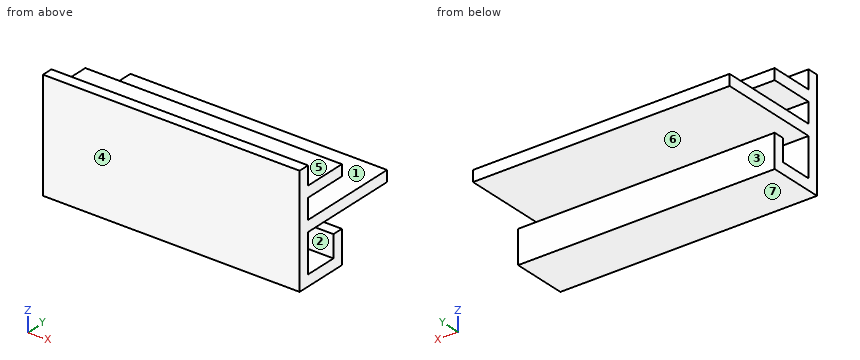
```python
from build123d import *

# Parameters (mm, degrees)
SKETCH_1_W      = 3
SKETCH_1_H      = 12
SKETCH_1_W_2    = 30
SKETCH_1_H_2    = 3
SKETCH_1_W_3    = 6
SKETCH_1_H_3    = 28
EXTRUDE_1_DEPTH = 70


with BuildPart() as part:
    # Sketch 1 → Extrude 1 (new body)
    with BuildSketch(Plane(origin=(0, 0, 0), x_dir=(0, 0, -1), z_dir=(1, 0, 0))):
        with Locations((-8.5, 7.5)):
            Rectangle(SKETCH_1_W, SKETCH_1_H)
        Rectangle(SKETCH_1_W_2, SKETCH_1_H_2)
        Polygon((15, 13.5), (12, 13.5), (12, 10.5), (12, 1.5), (15, 1.5), align=None)
        with Locations((9, 12)):
            Rectangle(SKETCH_1_W_3, SKETCH_1_H_2)
        with Locations((0, 15.5)):
            Rectangle(SKETCH_1_W, SKETCH_1_H_3)
    extrude(amount=EXTRUDE_1_DEPTH)


solid = part.part
```
CAD build for the part. Positions are in the model's coordinates, mm. Face numbers are marked on the shaded views. A direction names the side the tool comes from. Round coordinates to 2 decimals unless told otherwise and drop trailing zeros. Loops run counter-clockwise (first coordinate to the right, second up) from the corner with the lowest first, then second, coordinate; pieces in that order, holes last. Notation, with made-up numbers: M 32,77 L 53,77 A32 cw 53,107 Z; hole C -9.5,83 d8. An arc over 180 degrees is marked long. Return JSON: item names as keys, results as strings. Group by question number.
(1) Drop flat-ended pins along their axis: P1, Ø3, axis at x = 41.5, z = 5, coming from the +Y side; P2, Ø7, axis at x = 46, z = -8.5, coming from the +Y side; P3, Ø12, axis at x = 42, y = 25.5, coming from the +Z side. Give the stop position or say it passes through.
(2) Tool access for the marked faces 1, 2 and 3: list every direction of +Z, -Z, +X, -X, +Y, -Y with a clear straight run to the whole face (end or side of a thin tool).
(3) Mould opens along Z. For the marked faces 4, 5, 6 and 7 say: +Z half, -Z half, draft (parallel to the pull), parting line (faces both ways), or undercut.
(4) Saw through at D-D, the plane z = 4.75. List the corners of the cut face in (x, y), and give its area (3 significant figures).
(5) Saw through at A-A, the plane z = -7.75. List the corners of the cut face in (x, y), and give its area (3 significant figures).
(6) Saw through at C-C, the plane x = 8. List the corners of the cut face in (y, z), and give its area (3 significant figures).
(7) Wall check: probe 1 along Z at (x, y) = (33.5, 4.5); probe 2 along Y at (x, z) = (59.5, -8.5); probe 3 along Z at (x, y) = (25.5, 16). Give the ranges that are in metal, low to high. Write a range as [from, to].
(8) Saw through at B-B, the plane y = 8. List the corners of the cut face in (x, z), and give its area (3 significant figures).
Answer list:
{
 "1": {"P1": "y = 1.5", "P2": "y = 13.5", "P3": "z = 1.5"},
 "2": {"face 1": "+X, -X, +Y", "face 2": "+X, -X", "face 3": "-Z, +X, -X, +Y"},
 "3": {"face 4": "draft", "face 5": "+Z half", "face 6": "undercut", "face 7": "-Z half"},
 "4": {"outline": "M 0,-1.5 L 70,-1.5 L 70,1.5 L 0,1.5 Z", "area": "210 mm2"},
 "5": {"outline": "M 0,-1.5 L 70,-1.5 L 70,1.5 L 0,1.5 Z; M 0,10.5 L 70,10.5 L 70,13.5 L 0,13.5 Z", "area": "420 mm2"},
 "6": {"outline": "M -1.5,-15 L 13.5,-15 L 13.5,-6 L 10.5,-6 L 10.5,-12 L 1.5,-12 L 1.5,-1.5 L 29.5,-1.5 L 29.5,1.5 L 1.5,1.5 L 1.5,7 L 13.5,7 L 13.5,10 L 1.5,10 L 1.5,15 L -1.5,15 Z", "area": "264 mm2"},
 "7": {"probe 1": "[-15, -12], [-1.5, 1.5], [7, 10]", "probe 2": "[-1.5, 1.5], [10.5, 13.5]", "probe 3": "[-1.5, 1.5]"},
 "8": {"outline": "M 0,-15 L 70,-15 L 70,-12 L 0,-12 Z; M 0,-1.5 L 70,-1.5 L 70,1.5 L 0,1.5 Z; M 0,7 L 70,7 L 70,10 L 0,10 Z", "area": "630 mm2"}
}
